```python
from build123d import *

# Parameters (mm, degrees)
SKETCH1_W           = 26
SKETCH1_H           = 33
SKETCH1_R           = 5
SKETCH1_R_2         = 1.6
BOSS_EXTRUDE1_DEPTH = 3
FILLET2_R           = 3
SKETCH2_W           = 26
SKETCH2_H           = 3
BOSS_EXTRUDE2_DEPTH = 33
FILLET3_R           = 13
SKETCH3_R           = 4
SKETCH3_R_2         = 1.6
CUT_EXTRUDE1_DEPTH  = 3
FILLET4_R           = 2
FILLET5_R           = 1


with BuildPart() as part:
    # Sketch1 → Boss-Extrude1 (new body)
    with BuildSketch(Plane(origin=(0, 0, 0), x_dir=(1, 0, 0), z_dir=(0, 1, 0))):
        Rectangle(SKETCH1_W, SKETCH1_H)
        with Locations(Location((0, -0.5, 0), (0, 0, 270))):
            Circle(SKETCH1_R, mode=Mode.SUBTRACT)
        with Locations(Location((8, 6.5, 0), (0, 0, 270))):
            Circle(SKETCH1_R_2, mode=Mode.SUBTRACT)
        with Locations(Location((-8, 6.5, 0), (0, 0, 90))):
            Circle(SKETCH1_R_2, mode=Mode.SUBTRACT)
        with Locations(Location((8, -7.5, 0), (0, 0, 90))):
            Circle(SKETCH1_R_2, mode=Mode.SUBTRACT)
        with Locations(Location((-8, -7.5, 0), (0, 0, 270))):
            Circle(SKETCH1_R_2, mode=Mode.SUBTRACT)
    extrude(amount=BOSS_EXTRUDE1_DEPTH)

    # Fillet2
    fillet2_edges = [part.edges().sort_by_distance(p)[0] for p in [
        (13, 1.5, 16.5),
        (-13, 1.5, 16.5),
    ]]
    fillet(fillet2_edges, radius=FILLET2_R)

    # Sketch2 → Boss-Extrude2 (add)
    with BuildSketch(Plane(origin=(0, 3, 0), x_dir=(1, 0, 0), z_dir=(0, 1, 0))):
        with Locations((0, 15)):
            Rectangle(SKETCH2_W, SKETCH2_H)
    extrude(amount=BOSS_EXTRUDE2_DEPTH)

    # Fillet3
    fillet3_edges = [part.edges().sort_by_distance(p)[0] for p in [
        (-13, 36, -15),
        (13, 36, -15),
    ]]
    fillet(fillet3_edges, radius=FILLET3_R - 0.0001)  # a hair under: the kernel refuses the full size

    # Sketch3 → Cut-Extrude1 (cut)
    with BuildSketch(Plane.XY.offset(-13.5)):
        with Locations((0, 20)):
            Circle(SKETCH3_R)
        with Locations((8.5, 20)):
            Circle(SKETCH3_R_2)
        with Locations(Location((-8.5, 20, 0), (0, 0, 180))):
            Circle(SKETCH3_R_2)
    extrude(amount=-CUT_EXTRUDE1_DEPTH, mode=Mode.SUBTRACT)

    # Fillet4
    fillet4_edges = [part.edges().sort_by_distance(p)[0] for p in [
        (0, 0, -16.5),
    ]]
    fillet(fillet4_edges, radius=FILLET4_R)

    # Fillet5
    fillet5_edges = [part.edges().sort_by_distance(p)[0] for p in [
        (0, 3, -13.5),
    ]]
    fillet(fillet5_edges, radius=FILLET5_R)


solid = part.part
```
Read the model definition and answer for the solid it produces. Units are mm, in the model's axes. A direction names the side the tool comes from. Give positions to 0.01 mm unless a question says otherwise; leave off trailing zeros. Write each loop counter-clockwise with the first axis right and the second up, starting at its lowest first coordinate (ties: lowest second). Pieces come first, ordered by that corner, then holes. Notation, with made-up numbers: M 29,-3.5 L 37,-3.5 A16 ccw 37,21.5 Z; hole C 68.5,16 d9. An arc over 180 degrees is marked long. Put each result on its own line as item: value. Start each with the question number.
1. Which of the six approach directions +Z, -Z, +X, -X, +Y, -Y give full straight-line access (tool end or side, diameter ignored) to faces 1 (the cylindrical face through (0.18, 0.6, -15.93)), 2 (the flat face through (-3, 3, 5))?
2. For a pull along Z with two mould halves and no side action, classify faces 3 (the cylindrical face through (-0.521, 23.966, -14.979)), 4 (the cylindrical face through (12.1, 1.52, 15.64)), 5 (the cylindrical face through (8.97, 1.48, 8.77)) as released by +Z, released by -Z, zero draft, split by the parting line, or undercut.
3. Consider line 1 along X through (y, z) = (0.9, 7.5); line 2 along Y through (x, z) = (1.25, 8); line 3 along Z through (x, y) = (11, 26). Determine where each line is inside the solid, lowest interval first.
4. Each of these flat-tipped pins is pushed along its axis until it touches: pin 1 Ø3.5 at (x, z) = (8, 7.5) entering from -Y; pin 2 Ø5 at (x, z) = (8, -6.5) entering from +Y; pin 3 Ø5 at (x, y) = (0, 20) entering from +Z; pin 4 Ø1 at (x, y) = (9.5, 22.5) entering from +Z. Where does it stop, or does it pass through?
5. The part is cut by section B-B, the plane z = -7. Give the vertices of the cut face in (x, y), and give its area (3 significant figures).
6. The part is cut by section A-A, the plane y = 20. Give the vertices of the cut face in (x, z).
7. The part is cut by section D-D, the plane z = 0.5. Give the vertices of the cut face in (x, y), and give its area (3 significant figures).
8. The part is cut by section C-C, the plane x = 3.5. Give the vertices of the cut face in (y, z), and give its area (3 significant figures).
Final values:
1. face 1: -Z, +X, -X, -Y
1. face 2: +Z, +X, -X, +Y
2. face 3: zero draft
2. face 4: released by +Z
2. face 5: undercut
3. line 1: x = -13 to -9.6, -6.4 to 6.4, 9.6 to 13
3. line 2: y = 0 to 3
3. line 3: z = -16.5 to -13.5
4. pin 1: stops at y = 0
4. pin 2: stops at y = 3
4. pin 3: passes through
4. pin 4: stops at z = -13.5
5. outline: M -13,0 L -9.52,0 L -9.52,3 L -13,3 Z; M -6.48,0 L 6.48,0 L 6.48,3 L -6.48,3 Z; M 9.52,0 L 13,0 L 13,3 L 9.52,3 Z
5. area: 59.8 mm²
6. outline: M -13,-16.5 L -10.1,-16.5 L -10.1,-13.5 L -13,-13.5 Z; M -6.9,-16.5 L -4,-16.5 L -4,-13.5 L -6.9,-13.5 Z; M 4,-16.5 L 6.9,-16.5 L 6.9,-13.5 L 4,-13.5 Z; M 10.1,-16.5 L 13,-16.5 L 13,-13.5 L 10.1,-13.5 Z
7. outline: M -13,0 L -5,0 L -5,3 L -13,3 Z; M 5,0 L 13,0 L 13,3 L 5,3 Z
7. area: 48.0 mm²
8. outline: M 0,-14.5 A2 ccw 2,-16.5 L 18.06,-16.5 L 18.06,-13.5 L 4,-13.5 A1 cw 3,-12.5 L 3,-3.07 L 0,-3.07 Z; M 0,4.07 L 3,4.07 L 3,16.5 L 0,16.5 Z; M 21.94,-16.5 L 35.52,-16.5 L 35.52,-13.5 L 21.94,-13.5 Z
8. area: 163 mm²
